Read the model definition and answer for the solid it produces. Units are mm, in the model's axes. Round coordinates to 2 decimals unless told otherwise and drop trailing zeros. Loops run counter-clockwise (first coordinate to the right, second up) from the corner with the lowest first, then second, coordinate; pieces in that order, holes last. Notation, with made-up numbers: (45.5, -17) - (104.5, -17) arc R32 cw to (104.5, 11) - close; hole circle Ø5 at (7.5, 73.25). An arc over 180 degrees is marked (long way). Use CSV: the item, a comma, the result in double quotes. Start each with the question number.
1. Find section B-B (z = 73). Give the vertices of the cut face in (x, y).
2. Find section A-A (y = -56). Give the vertices of the cut face in (x, z).
3. Consider line 1 along X through (y, z) = (-57.7, 104); line 2 along Z through (x, y) = (-395.5, -55.95); line 3 along X through (y, z) = (-58.4, 218.5). Determine where each line is inside the solid, lowest interval first.
4. Given pin 1 Ø2.5 at (y, z) = (-56.5, 84.5) entering from -X; pin 2 Ø2.5 at (y, z) = (-57, 90) entering from +X, each flat-ended and moving along its own axis, determine where each tip first touches the part or whether it passes through.
Autodesk Inventor part; units mm, degrees
ref_plane "YZ Plane" through (0, 0, 0) normal (1, 0, 0) x (0, 1, 0)
ref_plane "XZ Plane" through (0, 0, 0) normal (0, 1, 0) x (-1, 0, 0)
ref_plane "XY Plane" through (0, 0, 0) normal (0, 0, 1) x (1, 0, 0)
sketch "Sketch1" plane through (0, 0, 0) normal (0, 0, 1) x (1, 0, 0)
  line L0 (185.4498, -59.7201) -> (-424.1502, -59.7201)
  line L1 (-424.1502, -59.7201) -> (-424.1502, -54.6401)
  line L2 (-424.1502, -54.6401) -> (185.4498, -54.6401)
  line L3 (185.4498, -54.6401) -> (185.4498, -59.7201)
  point P0 (0, 0)
  dimension "d0" = 609.6
  dimension "d1" = 5.08
extrude "Extrusion1" add sketch "Sketch1" along normal blind 228.6
sketch "Sketch2" plane through (-424.1502, -59.7201, 0) normal (0, -1, 0) x (1, 0, 0)
  line L0 (0, 0) -> (0, 228.6)
  line L1 (609.6, 0) -> (0, 0)
  line L2 (609.6, 0) -> (609.6, 228.6)
  line L3 (0, 228.6) -> (44.45, 228.6)
  line L4 (44.45, 228.6) -> (44.45, 177.8)
  line L5 (44.45, 177.8) -> (0, 177.8)
  line L6 (0, 177.8) -> (0, 228.6)
  line L7 (609.6, 228.6) -> (565.15, 228.6)
  line L8 (565.15, 228.6) -> (565.15, 177.8)
  line L9 (565.15, 177.8) -> (609.6, 177.8)
  line L10 (609.6, 177.8) -> (609.6, 228.6)
  line L11 (609.6, 60.96) -> (584.2, 60.96)
  line L12 (584.2, 60.96) -> (584.2, 143.51)
  line L13 (584.2, 143.51) -> (609.6, 143.51)
  line L14 (609.6, 143.51) -> (609.6, 60.96)
  line L15 (0, 60.96) -> (25.4, 60.96)
  line L16 (25.4, 60.96) -> (25.4, 143.51)
  line L17 (25.4, 143.51) -> (0, 143.51)
  line L18 (0, 143.51) -> (0, 60.96)
  point P0 (424.1502, 0)
  dimension "d4" = 44.45
  dimension "d5" = 50.8
  dimension "d6" = 44.45
  dimension "d7" = 50.8
  dimension "d8" = 60.96
  dimension "d9" = 60.96
  dimension "d10" = 25.4
  dimension "d11" = 25.4
  dimension "d12" = 82.55
  dimension "d13" = 82.55
extrude "Extrusion2" cut sketch "Sketch2" against normal blind 25.4
equation "\"d6\" = d4"
equation "\"d7\" = d5"
equation "\"d9\" = d8"
equation "\"d10\" = d11"
equation "\"d13\" = d12"
properties part number "ElectronicsBoardVerticalBottomDropped"
Filled sheet:
1,outline,"(-398.75, -59.72) - (160.05, -59.72) - (160.05, -54.64) - (-398.75, -54.64) - close"
2,outline,"(-424.15, 0) - (185.45, 0) - (185.45, 60.96) - (160.05, 60.96) - (160.05, 143.51) - (185.45, 143.51) - (185.45, 177.8) - (141, 177.8) - (141, 228.6) - (-379.7, 228.6) - (-379.7, 177.8) - (-424.15, 177.8) - (-424.15, 143.51) - (-398.75, 143.51) - (-398.75, 60.96) - (-424.15, 60.96) - close"
3,line 1,"x = -398.75 to 160.05"
3,line 2,"z = 0 to 177.8"
3,line 3,"x = -379.7 to 141"
4,pin 1,"stops at x = -398.75"
4,pin 2,"stops at x = 160.05"
